The model under review builds one solid part; all positions refer to its coordinate system, in mm. Face numbers are marked on the shaded views. A direction names the side the tool comes from. Coordinates: 2 decimals unless noted, no trailing zeros. Write each loop counter-clockwise with the first axis right and the second up, starting at its lowest first coordinate (ties: lowest second). Pieces come first, ordered by that corner, then holes.
```python
from build123d import *

# Parameters (mm, degrees)
SKETCH1_W               = 40.64
SKETCH1_H               = 50.8
BOSS_EXTRUDE1_DEPTH     = 12.7
CUT_EXTRUDE1_DEPTH      = 67.283780822
CUT_EXTRUDE1_DEPTH_BACK = 67.283780822
SKETCH3_W               = 16.502
SKETCH3_H               = 8.12
CUT_EXTRUDE2_DEPTH      = 67.283780822
CUT_EXTRUDE2_DEPTH_BACK = 67.283780822
SKETCH5_R               = 3.429
FILLET1_R               = 6.35


with BuildPart() as part:
    # Sketch1 → Boss-Extrude1 (new body)
    with BuildSketch(Plane(origin=(0, 0, 0), x_dir=(1, 0, 0), z_dir=(0, 1, 0))):
        with Locations((20.32, 25.4)):
            Rectangle(SKETCH1_W, SKETCH1_H)
    extrude(amount=BOSS_EXTRUDE1_DEPTH)

    # Sketch3 → Cut-Extrude1 (cut, two sides: drawn at the far end of the back side and taken through both)
    with BuildSketch(Plane(origin=(40.64, 0, 0), x_dir=(0, 0, -1), z_dir=(1, 0, 0)).offset(-CUT_EXTRUDE1_DEPTH_BACK)):
        with Locations((25.4, 8.89)):
            Rectangle(SKETCH3_W, SKETCH3_H)
    extrude(amount=CUT_EXTRUDE1_DEPTH + CUT_EXTRUDE1_DEPTH_BACK, mode=Mode.SUBTRACT)

    # Sketch5 → Cut-Extrude2 (cut, two sides: drawn at the far end of the back side and taken through both)
    with BuildSketch(Plane(origin=(0, 12.7, 0), x_dir=(1, 0, 0), z_dir=(0, 1, 0)).offset(-CUT_EXTRUDE2_DEPTH_BACK)):
        with Locations(Location((10.16, 8.636, 0), (0, 0, 270))):
            Circle(SKETCH5_R)
        with Locations(Location((30.48, 8.636, 0), (0, 0, 270))):
            Circle(SKETCH5_R)
        with Locations(Location((30.48, 42.164, 0), (0, 0, 270))):
            Circle(SKETCH5_R)
        with Locations(Location((10.16, 42.164, 0), (0, 0, 270))):
            Circle(SKETCH5_R)
    extrude(amount=CUT_EXTRUDE2_DEPTH + CUT_EXTRUDE2_DEPTH_BACK, mode=Mode.SUBTRACT)

    # Fillet1
    fillet1_edges = [part.edges().sort_by_distance(p)[0] for p in [
        (0, 6.35, -50.8),
        (40.64, 6.35, -50.8),
        (40.64, 6.35, 0),
        (0, 6.35, 0),
    ]]
    fillet(fillet1_edges, radius=FILLET1_R)


solid = part.part
```
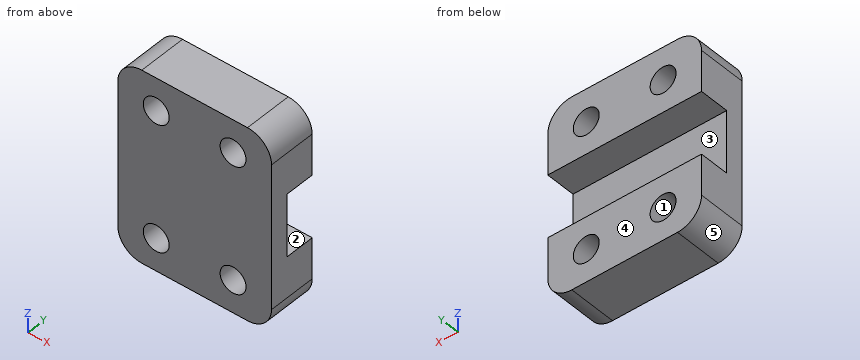
Item 1: Machinability: for the marked faces 1 and 2, which of the approach directions +Z, -Z, +X, -X, +Y, -Y give a long, thin tool a straight path to every point of the face, cutting with its end or side? Answer none if there is none.
Solved:
face 1: +Y, -Y
face 2: +X, -X, +Y
Item 2: To check wall thickness, follow line 1 along Z through (x, y) = (10.16, 8.25) (3 decimals); line 2 along Z through (x, y) = (30.48, 4.75) (3 decimals); line 3 along Z through (x, y) = (21, 9.25). State the ranges of each line that lie inside material, in increasing order.
Solved:
line 1: z = -50.8 to -45.593, -38.735 to -33.651, -17.149 to -12.065, -5.207 to 0
line 2: z = -50.8 to -45.593, -38.735 to -12.065, -5.207 to 0
line 3: z = -50.8 to -33.65, -17.15 to 0
Item 3: Mouldability with a two-part tool opening along Z and no side actions: class the marked faces 3, 4 and 5 as pulls with the +Z half, pulls with the -Z half, needs draft (parallel to the pull), parting line crosses it, or undercut.
Solved:
face 3: undercut
face 4: needs draft
face 5: pulls with the -Z half
Item 4: Take a section at D-D, the plane z = -29.5. Write out the cut boundary in (x, y).
Solved:
outline: (0, 0) - (40.64, 0) - (40.64, 4.83) - (0, 4.83) - close
Item 5: Take a section at C-C, the plane x = 18. Write out the cut boundary in (y, z).
Solved:
outline: (0, -50.8) - (12.7, -50.8) - (12.7, -33.65) - (4.83, -33.65) - (4.83, -17.15) - (12.7, -17.15) - (12.7, 0) - (0, 0) - close
Item 6: Take a section at A-A, the plane y = 3.5. Write out the cut boundary in (x, z) (3 decimals).
Solved:
outline: (0, -44.45) arc R6.35 ccw to (6.35, -50.8) - (34.29, -50.8) arc R6.35 ccw to (40.64, -44.45) - (40.64, -6.35) arc R6.35 ccw to (34.29, 0) - (6.35, 0) arc R6.35 ccw to (0, -6.35) - close; hole circle Ø6.858 at (10.16, -42.164); hole circle Ø6.858 at (10.16, -8.636); hole circle Ø6.858 at (30.48, -42.164); hole circle Ø6.858 at (30.48, -8.636)
Item 7: For pin 1 (5 mm diameter, centred on x = 16.5, z = -24.5, fed in from +Y); pin 2 (9 mm diameter, centred on x = 30.48, z = -42.164, fed in from +Y); pin 3 (5.5 mm diameter, centred on x = 10.16, z = -8.636, fed in from -Y), all flat-tipped, find the tip position at first contact; note any pin that passes through.
Solved:
pin 1: stops at y = 4.83
pin 2: stops at y = 12.7
pin 3: passes through
Item 8: Take a section at B-B, the plane x = 10.16. Write out the cut boundary in (y, z) (3 decimals), plus the area to 3 significant figures.
Solved:
outline: (0, -50.8) - (12.7, -50.8) - (12.7, -45.593) - (0, -45.593) - close; (0, -38.735) - (12.7, -38.735) - (12.7, -33.651) - (4.83, -33.651) - (4.83, -17.149) - (12.7, -17.149) - (12.7, -12.065) - (0, -12.065) - close; (0, -5.207) - (12.7, -5.207) - (12.7, 0) - (0, 0) - close
area: 341 mm2
